from build123d import *

# Parameters (mm, degrees)
F1_DEPTH = 30
F2_R     = 3.25
F3_DEPTH = 60.001


with BuildPart() as f1:
    # F0 (on Top) → F1 (new body)
    with BuildSketch(Plane.XY):
        with BuildLine():
            Line((-25, -1), (-25, -40))
            Line((-25, -40), (25, -40))
            Line((25, -40), (25, 20))
            Line((25, 20), (-25, 20))
            Line((-25, 20), (-25, 1))
            Line((-25, 1), (-12.459936, 1))
            ThreePointArc((-12.459936, 1), (-0.280101, 12.496861), (12.402618, 1.557262))
            ThreePointArc((12.402618, 1.557262), (1.278952, -12.434399), (-12.459936, -1))
            Line((-12.459936, -1), (-25, -1))
        make_face()
    extrude(amount=F1_DEPTH)

    # F2 (on face) → F3 (cut, through all)
    with BuildSketch(Plane.XZ.offset(40)):
        with Locations((-18, 15)):
            Circle(F2_R)
        with Locations((18, 15)):
            Circle(F2_R)
    extrude(amount=-F3_DEPTH, mode=Mode.SUBTRACT)


solid = f1.part
CAD build for the part. Positions are in the model's coordinates, mm. A direction names the side the tool comes from. Round coordinates to 2 decimals unless told otherwise and drop trailing zeros. Order: outer loops, then holes, each group sorted by start corner. A loop starts at its lowest first (then second) coordinate and runs counter-clockwise, first axis right, second up. Notation, with made-up numbers: (-8, 17.25) -> (32, 17.25) arc R19 cw to (32, 35.25) -> close; hole circle Ø8 at (81.25, 22). An arc over 180 degrees is marked (long way). Write item = value, one per line. Start each with the question number.
(1) Pull direction X, two halves, no side cores. Call faces 3 (the flat face through (0, -40, 15)), 4 (the cylindrical face through (-20.395, -20.773, 17.197)), 5 (the flat face through (25, -10, 15)): released by +X, released by -X, zero draft, split by the parting line, or undercut.
(2) Cut at B-B, the plane y = -3. List the corners of the cut face in (x, z), then the cut area to 3 significant figures.
(3) Probe line 1 (Z direction, x = -18, y = 7.5); line 2 (Y direction, x = 0, z = 21); line 3 (Y direction, x = -21.5, z = 5.75). List the from-to ranges inside material, lowest first. Write a range as [from, to].
(4) Cut at A-A, the plane x = 10. List the corners of the cut face in (y, z).
(5) Which spindle directions (+Z, -Z, +X, -X, +Y, -Y) get a long thin tool onto all of the face, cutting with end or side? Do faces 1 (the flat face through (0, -16, 30)), 2 (the flat face through (-22, 1, 15)). Say none if no direction does.
(6) Cut at C-C, the plane z = 15. List the corners of the cut face in (x, y), then the cut area to 3 significant figures.
(7) Pin check, flat tip, straight feed: P1, Ø4, axis at x = -18, z = 15, coming from the +Y side. Stop position of the tip, or through.
(8) Cut at D-D, the plane x = -18. List the corners of the cut face in (y, z).
Model answer:
q1.face_3 = zero draft
q1.face_4 = undercut
q1.face_5 = released by +X
q2.outline = (-25, 0) -> (-12.13, 0) -> (-12.13, 30) -> (-25, 30) -> close; (12.13, 0) -> (25, 0) -> (25, 30) -> (12.13, 30) -> close; hole circle Ø6.5 at (-18, 15); hole circle Ø6.5 at (18, 15)
q2.area = 706 mm2
q3.line_1 = [0, 11.75], [18.25, 30]
q3.line_2 = [-40, -12.5], [12.5, 20]
q3.line_3 = [-40, -1], [1, 20]
q4.outline = (-40, 0) -> (-7.5, 0) -> (-7.5, 30) -> (-40, 30) -> close; (7.5, 0) -> (20, 0) -> (20, 30) -> (7.5, 30) -> close
q5.face_1 = +Z, +X, -X, +Y, -Y
q5.face_2 = +Z, -Z, -X
q6.outline = (-25, -40) -> (-21.25, -40) -> (-21.25, -1) -> (-25, -1) -> close; (-25, 1) -> (-21.25, 1) -> (-21.25, 20) -> (-25, 20) -> close; (-14.75, -40) -> (14.75, -40) -> (14.75, 20) -> (-14.75, 20) -> (-14.75, 1) -> (-12.46, 1) arc R12.5 cw (long way) to (-12.46, -1) -> (-14.75, -1) -> close; (21.25, -40) -> (25, -40) -> (25, 20) -> (21.25, 20) -> close
q6.area = 1,720 mm2
q7.P1 = through
q8.outline = (-40, 0) -> (-1, 0) -> (-1, 11.75) -> (-40, 11.75) -> close; (-40, 18.25) -> (-1, 18.25) -> (-1, 30) -> (-40, 30) -> close; (1, 0) -> (20, 0) -> (20, 11.75) -> (1, 11.75) -> close; (1, 18.25) -> (20, 18.25) -> (20, 30) -> (1, 30) -> close
